Check sheet for the modelled part. Datum: model origin and axes. Units: mm. Round coordinates to 2 decimals unless told otherwise and drop trailing zeros. Loops run counter-clockwise (first coordinate to the right, second up) from the corner with the lowest first, then second, coordinate; pieces in that order, holes last. Notation, with made-up numbers: (-39, 41.25) - (-12, 41.25) arc R31 ccw to (-12, 75.25) - close; hole circle Ø10 at (41.25, -29.75). An arc over 180 degrees is marked (long way). Put each result on its own line as item: value. Start each with the question number.
Item 1: Draft check along X on faces 1 (the cylindrical face through (-29.97, -1.97, -1.32)), 2 (the conical face through (14.92, -2.2, 17.36)), 3 (the flat face through (0, 0, 20)). Enter one of: pulls with the +X half, pulls with the -X half, needs draft (parallel to the pull), parting line crosses it, or undercut.
Item 2: Gauge pin test, flat ends, axial feed: pin 1 Ø3.5 at (x, z) = (26, 0) entering from +Y; pin 2 Ø1 at (y, z) = (-3, -10.5) entering from +X; pin 3 Ø1.5 at (x, y) = (21.5, -1) entering from +Z; pin 4 Ø3 at (x, z) = (-26, 0) entering from -Y. Record the tip position at first contact, or that the pin passes through.
Item 3: Section check D-D, the plane z = -26. Record the cut outline in (x, y).
Item 4: Section check A-A, the plane y = -1.3. Give the number of separate pieces and of enclosed holes in the cut face, and give its area (3 significant figures).
Item 5: Section check C-C, the plane z = 0. Record the cut outline in (x, y), and give its area (3 significant figures).
Item 6: Material ranges on line 1 along Z through (x, y) = (0, -1.4); line 2 along Z through (x, y) = (16, -3.05), recorded low to high.
Item 7: Section check B-B, the plane x = -4. Record the cut outline in (y, z).
from build123d import *

# Parameters (mm, degrees)
SKETCH1_R                                           = 30
BOSS_EXTRUDE1_DEPTH                                 = 4
SKETCH8_R                                           = 15.5
CUT_EXTRUDE1_DEPTH                                  = 6
CSK_FOR_M3_COUNTERSUNK_FLAT_HEAD_SCR_2_COUNT        = 2
CSK_FOR_M3_COUNTERSUNK_FLAT_HEAD_SCR_2_PITCH        = 31
CSK_FOR_M3_COUNTERSUNK_FLAT_HEAD_SCR_3_COUNT        = 2
CSK_FOR_M3_COUNTERSUNK_FLAT_HEAD_SCR_3_PITCH        = 43.840620434
CSK_FOR_M3_COUNTERSUNK_FLAT_HEAD_SCR_4_COUNT        = 2
CSK_FOR_M3_COUNTERSUNK_FLAT_HEAD_SCR_4_PITCH        = 31
CSK_FOR_M3_COUNTERSUNK_FLAT_HEAD_SCREW3_D           = 3.2
CSK_FOR_M3_COUNTERSUNK_FLAT_HEAD_SCREW3_CSINK_D     = 6.3
CSK_FOR_M3_COUNTERSUNK_FLAT_HEAD_SCREW3_CSINK_ANGLE = 90


with BuildPart() as part:
    # Sketch1 → Boss-Extrude1 (new body)
    with BuildSketch(Plane(origin=(0, 0, 0), x_dir=(1, 0, 0), z_dir=(0, 1, 0))):
        Circle(SKETCH1_R)
    extrude(amount=-BOSS_EXTRUDE1_DEPTH)

    # Sketch8 → Cut-Extrude1 (cut)
    with BuildSketch(Plane.XZ.offset(4)):
        Circle(SKETCH8_R)
    extrude(amount=-CUT_EXTRUDE1_DEPTH, mode=Mode.SUBTRACT)

    # Sketch16 → CSK for M3 Countersunk Flat Head Screw2 (revolve, cut)
    with BuildSketch(Plane(origin=(15.5, 0, 15.5), x_dir=(0, 0, 1), z_dir=(1, 0, 0))):
        Polygon((0, 0), (0, 4), (1.8, 4), (1.8, 2.35), (4.15, 0), align=None)
    csk_for_m3_countersunk_flat_head_screw2 = revolve(axis=Axis((15.5, 6.35, 15.5), (0, -1, 0)), mode=Mode.SUBTRACT)

    # CSK for M3 Countersunk Flat Head Scr 2: CSK for M3 Countersunk Flat Head Screw2 ×2
    with Locations(*[(0, 0, -i * CSK_FOR_M3_COUNTERSUNK_FLAT_HEAD_SCR_2_PITCH) for i in range(1, CSK_FOR_M3_COUNTERSUNK_FLAT_HEAD_SCR_2_COUNT)]):
        add(csk_for_m3_countersunk_flat_head_screw2, mode=Mode.SUBTRACT)

    # CSK for M3 Countersunk Flat Head Scr 3: CSK for M3 Countersunk Flat Head Screw2 ×2
    with Locations(*[Vector(-0.707106781, 0, -0.707106781) * (i * CSK_FOR_M3_COUNTERSUNK_FLAT_HEAD_SCR_3_PITCH) for i in range(1, CSK_FOR_M3_COUNTERSUNK_FLAT_HEAD_SCR_3_COUNT)]):
        add(csk_for_m3_countersunk_flat_head_screw2, mode=Mode.SUBTRACT)

    # CSK for M3 Countersunk Flat Head Scr 4: CSK for M3 Countersunk Flat Head Screw2 ×2
    with Locations(*[(-i * CSK_FOR_M3_COUNTERSUNK_FLAT_HEAD_SCR_4_PITCH, 0, 0) for i in range(1, CSK_FOR_M3_COUNTERSUNK_FLAT_HEAD_SCR_4_COUNT)]):
        add(csk_for_m3_countersunk_flat_head_screw2, mode=Mode.SUBTRACT)

    # CSK for M3 Countersunk Flat Head Screw3 (through all)
    with Locations(Plane.XZ.offset(4)):
        with Locations((0, 26), (26, 0), (0, -26), (-26, 0)):
            CounterSinkHole(CSK_FOR_M3_COUNTERSUNK_FLAT_HEAD_SCREW3_D / 2, CSK_FOR_M3_COUNTERSUNK_FLAT_HEAD_SCREW3_CSINK_D / 2, counter_sink_angle=CSK_FOR_M3_COUNTERSUNK_FLAT_HEAD_SCREW3_CSINK_ANGLE)


solid = part.part
Check result:
1. face 1: parting line crosses it
1. face 2: undercut
1. face 3: needs draft
2. pin 1: y = 0
2. pin 2: x = 28.28
2. pin 3: z = 21.67
2. pin 4: through
3. outline: (-14.97, -4) - (-3.15, -4) - (-1.6, -2.45) - (-1.6, 0) - (-14.97, 0) - close; (1.6, -2.45) - (3.15, -4) - (14.97, -4) - (14.97, 0) - (1.6, 0) - close
4. separate pieces: 1
4. enclosed holes: 9
4. area: 1,940 mm²
5. outline: (-30, -4) - (-29.15, -4) - (-27.6, -2.45) - (-27.6, 0) - (-30, 0) - close; (-24.4, -2.45) - (-22.85, -4) - (-15.5, -4) - (-15.5, 0) - (-24.4, 0) - close; (15.5, -4) - (22.85, -4) - (24.4, -2.45) - (24.4, 0) - (15.5, 0) - close; (27.6, -2.45) - (29.15, -4) - (30, -4) - (30, 0) - (27.6, 0) - close
5. area: 85.6 mm²
6. line 1: -30 to -27.6, -24.4 to -15.5, 15.5 to 24.4, 27.6 to 30
6. line 2: -25.38 to -17.23, -13.77 to 13.77, 17.23 to 25.38
7. outline: (-4, -29.73) - (0, -29.73) - (0, -14.97) - (-4, -14.97) - close; (-4, 14.97) - (0, 14.97) - (0, 29.73) - (-4, 29.73) - close
